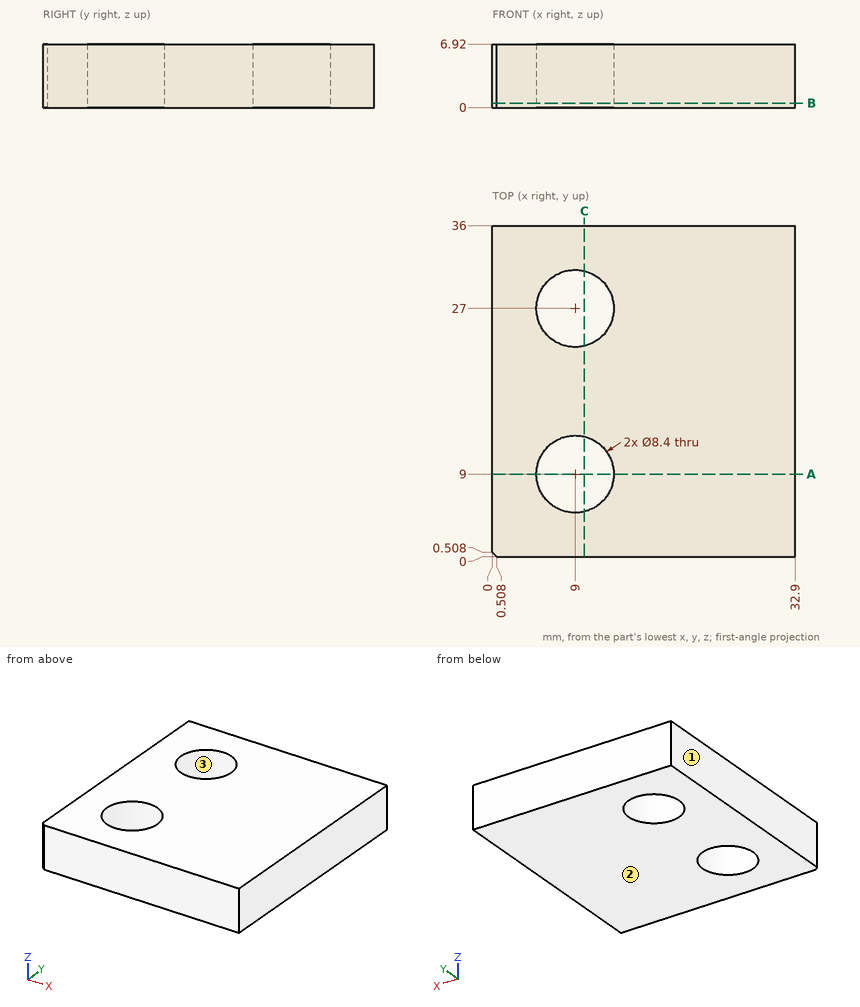
Could you check a few things on this drawing? It's one solid part, dimensions in mm from its lowest x, y, z. Coordinates: 2 decimals unless noted, no trailing zeros. Order: outer loops, then holes, each group sorted by start corner. A loop starts at its lowest first (then second) coordinate and runs counter-clockwise, first axis right, second up.
1. Thinking about a two-plate mould opening in X: for the marked faces 1, 2 and 3, which applies, +X half, -X half, draft (parallel to the pull), parting line (faces both ways), or undercut?
2. If we section it at C-C (x = 10): Please give me the cut outline in (y, z).
3. If we section it at A-A (y = 9): Please give me the cut outline in (x, z).
4. I need wall thicknesses on line 1 (Y direction, x = 9, z = 1.5); line 2 (X direction, y = 28, z = 3); line 3 (Y direction, x = 5.5, z = 6). Which ranges of each line are inside material? Lowest first, please.
5. If we section it at B-B (z = 0.5): Please give me the cut outline in (x, y), then the cut area to 3 significant figures.
Entries:
1. face 1: -X half
1. face 2: draft
1. face 3: undercut
2. outline: (0, 0) - (4.92, 0) - (4.92, 6.92) - (0, 6.92) - close; (13.08, 0) - (22.92, 0) - (22.92, 6.92) - (13.08, 6.92) - close; (31.08, 0) - (36, 0) - (36, 6.92) - (31.08, 6.92) - close
3. outline: (0, 0) - (4.8, 0) - (4.8, 6.92) - (0, 6.92) - close; (13.2, 0) - (32.9, 0) - (32.9, 6.92) - (13.2, 6.92) - close
4. line 1: y = 0 to 4.8, 13.2 to 22.8, 31.2 to 36
4. line 2: x = 0 to 4.92, 13.08 to 32.9
4. line 3: y = 0 to 6.68, 11.32 to 24.68, 29.32 to 36
5. outline: (0, 0.51) - (0.51, 0) - (32.9, 0) - (32.9, 36) - (0, 36) - close; hole circle Ø8.4 at (9, 9); hole circle Ø8.4 at (9, 27)
5. area: 1,070 mm2
